```python
from build123d import *

# Parameters (mm, degrees)
F1_DEPTH = 25.4
F2_R     = 2.54


with BuildPart() as f1:
    # F0 (on Top) → F1 (new body)
    with BuildSketch(Plane.XY):
        with BuildLine():
            Line((-79.014186, 78.602763), (-100.253638, 78.602763))
            Line((-100.253638, 78.602763), (-100.253638, 0))
            ThreePointArc((-100.253638, 0), (-112.683548, -12.42991), (-125.113457, 0))
            Line((-125.113457, 0), (-141.525768, 0))
            ThreePointArc((-141.525768, 0), (-110.269977, -31.255791), (-79.014186, 0))
            Line((-79.014186, 0), (-79.014186, 78.602763))
        make_face()
    extrude(amount=F1_DEPTH)

    # F2
    f2_edges = [f1.edges().sort_by_distance(p)[0] for p in [
        (-79.014186, 39.301381, 25.4),
        (-89.633912, 78.602763, 25.4),
        (-100.253638, 39.301381, 25.4),
        (-112.683548, -12.42991, 25.4),
        (-133.319613, 0, 25.4),
        (-110.269977, -31.255791, 25.4),
        (-79.014186, 39.301381, 0),
        (-89.633912, 78.602763, 0),
        (-100.253638, 39.301381, 0),
        (-112.683548, -12.42991, 0),
        (-133.319613, 0, 0),
        (-110.269977, -31.255791, 0),
        (-79.014186, 78.602763, 12.7),
        (-100.253638, 78.602763, 12.7),
        (-125.113457, 0, 12.7),
        (-141.525768, 0, 12.7),
    ]]
    fillet(f2_edges, radius=F2_R)


solid = f1.part
```
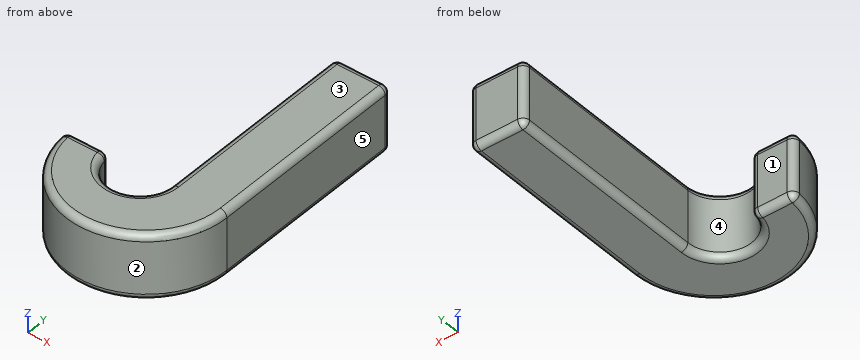
Can you work these out from the model? Positions are in its coordinate system, mm. Face numbers are marked on the shaded views. A direction names the side the tool comes from. Coordinates: 2 decimals unless noted, no trailing zeros. Write each loop counter-clockwise with the first axis right and the second up, starting at its lowest first coordinate (ties: lowest second). Pieces come first, ordered by that corner, then holes. Notation, with made-up numbers: M -19.75,69 L 21.25,69 A25 cw 21.25,100 Z; hole C -1,-39.5 d10. An arc over 180 degrees is marked long. Answer as CSV lines item,"result".
Item 1: Imagine slicing it at C-C on z = 1.5. List the corners of the cut face in (x, y) for me, plus the area to 3 significant figures.
Geometry results:
outline,"M -141.18,-2.74 A31.03 ccw -79.24,0 L -79.24,76.06 A2.32 ccw -81.55,78.38 L -97.71,78.38 A2.32 ccw -100.03,76.06 L -100.03,0 A12.65 cw -125.15,-2.15 A2.32 ccw -127.44,-0.22 L -138.87,-0.22 A2.32 ccw Z"
area,"2,880 mm2"
Item 2: Please list where these lines run through material, in increasing order: line 1 along X through (y, z) = (-0.5, 15.5); line 2 along X through (y, z) = (8, 10.75); line 3 along X through (y, z) = (-9.5, 1.75).
Geometry results:
line 1,"x = -140.39 to -125.92, -100.26 to -79.02"
line 2,"x = -100.25 to -79.01"
line 3,"x = -139.91 to -120.89, -104.47 to -80.63"
Item 3: Imagine slicing it at B-B on y = 59. List the corners of the cut face in (x, z) for me.
Geometry results:
outline,"M -100.25,2.54 A2.54 ccw -97.71,0 L -81.55,0 A2.54 ccw -79.01,2.54 L -79.01,22.86 A2.54 ccw -81.55,25.4 L -97.71,25.4 A2.54 ccw -100.25,22.86 Z"
Item 4: Imagine slicing it at A-A on z = 16.25. List the corners of the cut face in (x, y) for me.
Geometry results:
outline,"M -141.4,-2.76 A31.26 ccw -79.01,0 L -79.01,76.06 A2.54 ccw -81.55,78.6 L -97.71,78.6 A2.54 ccw -100.25,76.06 L -100.25,0 A12.43 cw -124.93,-2.11 A2.54 ccw -127.44,0 L -138.87,0 A2.54 ccw Z"
Item 5: We'd pull the mould along X, two halves only. Please class the marked faces 3, 4 and 5: +X half, -X half, draft (parallel to the pull), parting line (faces both ways), or undercut.
Geometry results:
face 3,"draft"
face 4,"undercut"
face 5,"+X half"
Item 6: I'm going to push flat-ended pins straight in: P1, Ø2, axis at x = -134, z = 20.5, coming from the +Y side; P2, Ø4, axis at x = -106.5, z = 10, coming from the +Y side; P3, Ø1, axis at y = 18.5, z = 14, coming from the -X side. Where does each tip first touch, or does it pass through?
Geometry results:
P1,"stops at y = 0"
P2,"stops at y = -9.36"
P3,"stops at x = -100.25"
Item 7: On a 3-axis mill with a long thin cutter (end or side, diameter ignored), from which of +Z, -Z, +X, -X, +Y, -Y can I reach the whole of each face in a straight line? I mean the marked faces 1 and 2. Say none if no direction works.
Geometry results:
face 1,"+Z, -Z, -X, +Y"
face 2,"+Z, -Z, -Y"
